Verification items for this drawing (mm, ordinates from the low corner). A direction names the side the tool comes from. Round coordinates to 2 decimals unless told otherwise and drop trailing zeros. Loops run counter-clockwise (first coordinate to the right, second up) from the corner with the lowest first, then second, coordinate; pieces in that order, holes last. Notation, with made-up numbers: (56.5, -36.75) -> (110.5, -36.75) arc R23 ccw to (110.5, -17.75) -> close; hole circle Ø10 at (67, 21.5). An arc over 180 degrees is marked (long way). One line per question, with ' | ' between items.
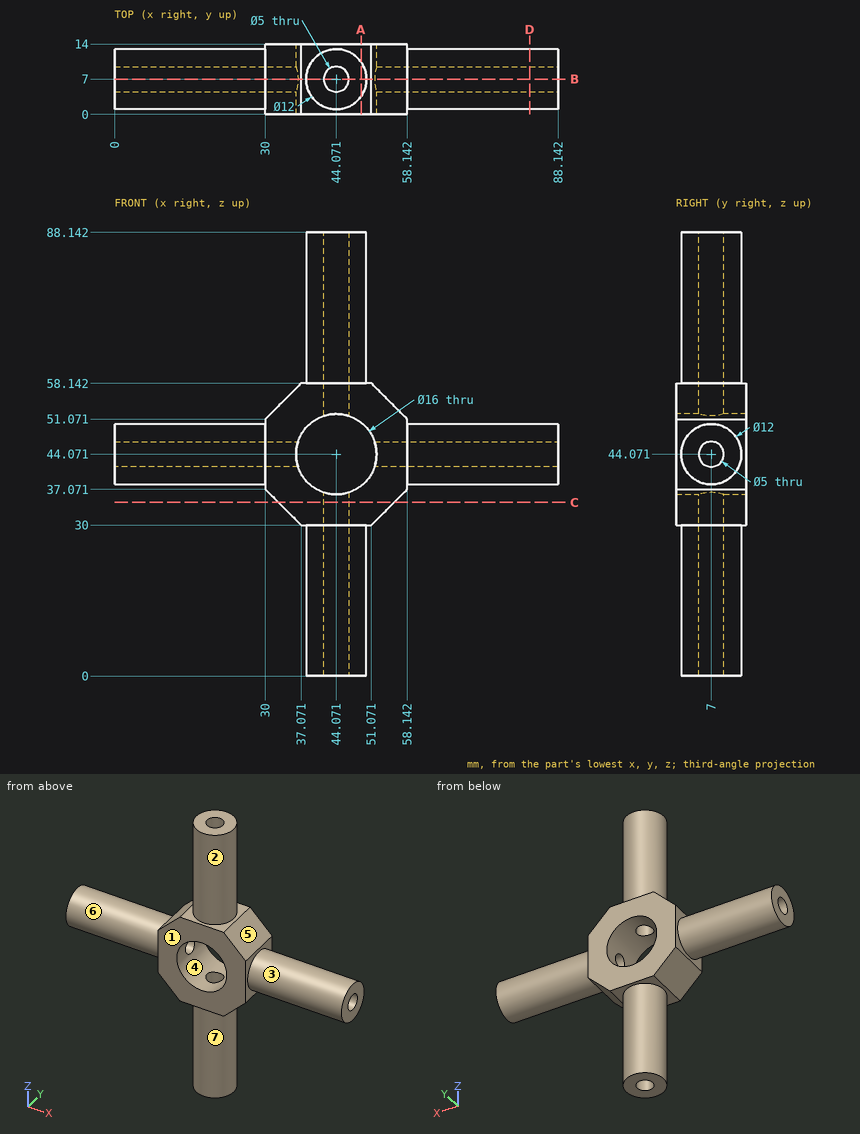
(1) Sectioned sample at C-C, the plane z = 34.5. Record the cut outline in (x, y).
Answer:
outline: (32.57, 0) -> (55.57, 0) -> (55.57, 14) -> (32.57, 14) -> close; hole circle Ø5 at (44.07, 7)
(2) Scan lines: probe 1 along Z at (x, y) = (44.5, 3); probe 2 along Y at (x, z) = (46, 60.5); probe 3 along X at (y, z) = (5, 77) (1 decimal). Record each from-to range of solid material in increasing order.
Answer:
probe 1: z = 0 to 36.08, 52.06 to 88.14 | probe 2: y = 1.32 to 5.41, 8.59 to 12.68 | probe 3: x = 38.4 to 42.6, 45.6 to 49.7
(3) Mould release check, pull along Z, two halves, no side actions. Record for the marked faces 4, 5, 6 and 7: +Z half, -Z half, draft (parallel to the pull), parting line (faces both ways), or undercut.
Answer:
face 4: undercut | face 5: +Z half | face 6: parting line | face 7: draft
(4) Go/stop test with flat-tipped pins: pin 1 (2 mm diameter, centred on x = 70, y = 12, fed in from +Z); pin 2 (12 mm diameter, centred on x = 39.5, z = 67.5, fed in from -Y); pin 3 (6 mm diameter, centred on y = 8.5, z = 76, fed in from -X). Record where each tip stops, or that it passes through.
Answer:
pin 1: stops at z = 48.54 | pin 2: stops at y = 1 | pin 3: stops at x = 38.07
(5) Set-up check for the marked faces 1, 2 and 3: record each of +Z, -Z, +X, -X, +Y, -Y from which the full face is reachable in a straight line by a thin tool's end or side.
Answer:
face 1: +Z, -Z, +X, -X, -Y | face 2: +Z | face 3: +X
(6) Sectioned sample at D-D, the plane x = 82.5. Record the cut outline in (y, z).
Answer:
outline: circle Ø12 at (7, 44.07); hole circle Ø5 at (7, 44.07)
(7) Sectioned sample at B-B, the plane y = 7. Count the separate pieces of the cut face and the enclosed holes in it, and give its area (3 significant figures).
Answer:
separate pieces: 4 | enclosed holes: 0 | area: 1,210 mm2
(8) Sectioned sample at A-A, the plane x = 49. Record the cut outline in (y, z), and give its area (3 significant figures).
Answer:
outline: (0, 30) -> (3.58, 30) -> (3.58, 0) -> (10.42, 0) -> (10.42, 30) -> (14, 30) -> (14, 37.77) -> (0, 37.77) -> close; (0, 50.37) -> (14, 50.37) -> (14, 58.14) -> (10.42, 58.14) -> (10.42, 88.14) -> (3.58, 88.14) -> (3.58, 58.14) -> (0, 58.14) -> close | area: 628 mm2
